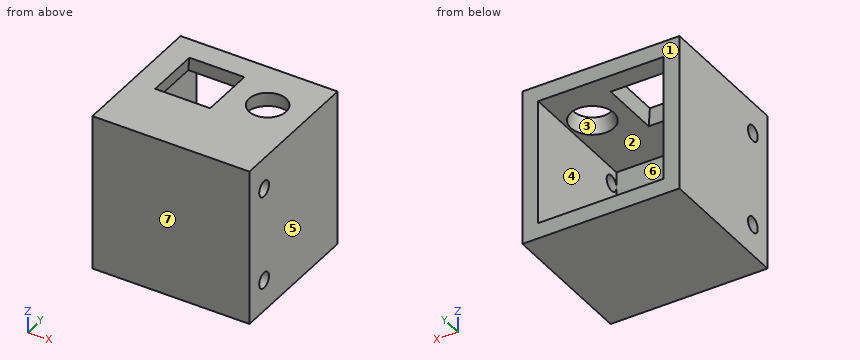
from build123d import *

# Parameters (mm, degrees)
ESQUISSE1_W                       = 10
ESQUISSE1_H                       = 10
BOSS_EXTRU_1_DEPTH                = 9
ESQUISSE3_R                       = 1.18058501
ENL_V_MAT_EXTRU_3_DEPTH           = 1.25
ENL_V_MAT_EXTRU_3_DRAFT           = 11
ESQUISSE3_W                       = 3.5
ESQUISSE3_H                       = 3.5
ENL_V_MAT_EXTRU_3_PROFILE_2_DEPTH = 1.25
ENL_V_MAT_EXTRU_3_PROFILE_2_DRAFT = 11
ESQUISSE5_W                       = 8
ESQUISSE5_H                       = 8
ENL_V_MAT_EXTRU_4_DEPTH           = 8
ESQUISSE7_R                       = 0.5
ENL_V_MAT_EXTRU_5_DEPTH           = 17.763054614


with BuildPart() as part:
    # Esquisse1 → Boss.-Extru.1 (new body)
    with BuildSketch(Plane(origin=(0, 0, 0), x_dir=(1, 0, 0), z_dir=(0, 1, 0))):
        with Locations((5, 5)):
            Rectangle(ESQUISSE1_W, ESQUISSE1_H)
    extrude(amount=BOSS_EXTRU_1_DEPTH)


with BuildPart() as enl_v_mat_extru_3_tool:
    # Esquisse3 → Enlèv. mat.-Extru.3 (with draft: the straight prism first)
    with BuildSketch(Plane.XY):
        with Locations((7.481483156, 5.897810635)):
            Circle(ESQUISSE3_R)
    extrude(amount=-ENL_V_MAT_EXTRU_3_DEPTH)
    # Enlèv. mat.-Extru.3: the draft: its side faces are tilted about the plane it starts from
    enl_v_mat_extru_3_sides = [enl_v_mat_extru_3_tool.faces().sort_by_distance(p)[0] for p in [
        (6.300898146, 5.897810635, -0.625),
    ]]
    draft(enl_v_mat_extru_3_sides, Plane.XY, ENL_V_MAT_EXTRU_3_DRAFT)


with BuildPart() as part_1:
    add(part.part)

    # Enlèv. mat.-Extru.3: cut by enl_v_mat_extru_3_tool
    add(enl_v_mat_extru_3_tool.part, mode=Mode.SUBTRACT)


with BuildPart() as enl_v_mat_extru_3_profile_2_tool:
    # Esquisse3 → Enlèv. mat.-Extru.3 profile 2 (with draft: the straight prism first)
    with BuildSketch(Plane.XY):
        with Locations((3.25, 5.75)):
            Rectangle(ESQUISSE3_W, ESQUISSE3_H)
    extrude(amount=-ENL_V_MAT_EXTRU_3_PROFILE_2_DEPTH)
    # Enlèv. mat.-Extru.3 profile 2: the draft: its side faces are tilted about the plane it starts from
    enl_v_mat_extru_3_profile_2_sides = [enl_v_mat_extru_3_profile_2_tool.faces().sort_by_distance(p)[0] for p in [
        (1.5, 5.75, -0.625),
        (3.25, 4, -0.625),
        (5, 5.75, -0.625),
        (3.25, 7.5, -0.625),
    ]]
    draft(enl_v_mat_extru_3_profile_2_sides, Plane.XY, ENL_V_MAT_EXTRU_3_PROFILE_2_DRAFT)


with BuildPart() as part_2:
    add(part_1.part)

    # Enlèv. mat.-Extru.3 profile 2: cut by enl_v_mat_extru_3_profile_2_tool
    add(enl_v_mat_extru_3_profile_2_tool.part, mode=Mode.SUBTRACT)

    # Esquisse5 → Enlèv. mat.-Extru.4 (cut)
    with BuildSketch(Plane(origin=(0, 9, 0), x_dir=(1, 0, 0), z_dir=(0, 1, 0))):
        with Locations((5, 5)):
            Rectangle(ESQUISSE5_W, ESQUISSE5_H)
    extrude(amount=-ENL_V_MAT_EXTRU_4_DEPTH, mode=Mode.SUBTRACT)

    # Esquisse7 → Enlèv. mat.-Extru.5 (cut, through all)
    with BuildSketch(Plane(origin=(10, 0, 0), x_dir=(0, 0, -1), z_dir=(1, 0, 0))):
        with Locations((2, 1.5)):
            Circle(ESQUISSE7_R)
        with Locations((8, 1.5)):
            Circle(ESQUISSE7_R)
    extrude(amount=-ENL_V_MAT_EXTRU_5_DEPTH, mode=Mode.SUBTRACT)


solid = part_2.part
Work out the finished part from the listing and answer in its coordinate system (mm). Face numbers are marked on the shaded views. A direction names the side the tool comes from. Give positions to 0.01 mm unless a question says otherwise; leave off trailing zeros. Loops run counter-clockwise (first coordinate to the right, second up) from the corner with the lowest first, then second, coordinate; pieces in that order, holes last. Notation, with made-up numbers: (3.5, 43.25) -> (56.5, 43.25) arc R15 ccw to (56.5, 65.25) -> close; hole circle Ø2 at (63.5, -11.75). An arc over 180 degrees is marked (long way). Use a Markdown table: item, result. Add a question column.
1) The part is cut by section B-B, the plane y = 1.5. Determine the outline of the cut face in (x, z), plus the area to 3 significant figures.
2) Consider line 1 along Z through (x, y) = (9.65, 1.5); line 2 along Z through (x, y) = (5.5, 8.5); line 3 along X through (y, z) = (6.75, -4). Determine where each line is inside the solid, lowest interval first.
3) The part is cut by section C-C, the plane z = -3.5. Determine the outline of the cut face in (x, y).
4) The part is cut by section A-A, the plane x = 2.25. Determine the outline of the cut face in (y, z), plus the area to 3 significant figures.
5) This flat-tipped pin is pushed along its axis until it touches: P1, Ø2.5, axis at x = 3, y = 6, coming from the +Z side. Where does it stop, or does it pass through?
6) For a pull along X with two mould halves and no side action, classify the marked faces 4, 5, 6 and 7 as +X half, -X half, draft (parallel to the pull), parting line (faces both ways), or undercut.
7) Which of the six approach directions +Z, -Z, +X, -X, +Y, -Y give full straight-line access (tool end or side, diameter ignored) to the marked faces 1, 2 and 3?
8) The part is cut by section D-D, the plane y = 4.25. Determine the outline of the cut face in (x, z), plus the area to 3 significant figures.
Reported:
| question | item | result |
|---|---|---|
| 1 | outline | (0, -10) -> (10, -10) -> (10, -8.5) -> (9, -8.5) -> (9, -9) -> (1, -9) -> (1, -8.5) -> (0, -8.5) -> close; (0, -7.5) -> (1, -7.5) -> (1, -2.5) -> (0, -2.5) -> close; (0, -1.5) -> (1, -1.5) -> (1, -1) -> (9, -1) -> (9, -1.5) -> (10, -1.5) -> (10, 0) -> (0, 0) -> close; (9, -7.5) -> (10, -7.5) -> (10, -2.5) -> (9, -2.5) -> close |
| 1 | area | 32.0 mm^2 |
| 2 | line 1 | z = -10 to -8.5, -7.5 to -2.5, -1.5 to 0 |
| 2 | line 2 | z = -10 to -9, -1 to 0 |
| 2 | line 3 | x = 0 to 1, 9 to 10 |
| 3 | outline | (0, 0) -> (10, 0) -> (10, 9) -> (9, 9) -> (9, 1) -> (1, 1) -> (1, 9) -> (0, 9) -> close |
| 4 | outline | (0, -10) -> (9, -10) -> (9, -9) -> (1, -9) -> (1, -1) -> (3.81, -1) -> (4, 0) -> (0, 0) -> close; (7.5, 0) -> (7.69, -1) -> (9, -1) -> (9, 0) -> close |
| 4 | area | 22.3 mm^2 |
| 5 | P1 | stops at z = -9 |
| 6 | face 4 | undercut |
| 6 | face 5 | +X half |
| 6 | face 6 | undercut |
| 6 | face 7 | draft |
| 7 | face 1 | +Z, -Z, +X, -X, +Y |
| 7 | face 2 | +Y |
| 7 | face 3 | none |
| 8 | outline | (0, -10) -> (10, -10) -> (10, 0) -> (5, 0) -> (5.19, -1) -> (9, -1) -> (9, -9) -> (1, -9) -> (1, -1) -> (1.31, -1) -> (1.5, 0) -> (0, 0) -> close |
| 8 | area | 32.3 mm^2 |
